Here's how the part is built. I have some questions about the finished solid (model axes, mm). Face numbers are marked on the shaded views. A direction names the side the tool comes from. Round coordinates to 2 decimals unless told otherwise and drop trailing zeros. Use a Markdown table: item, result.
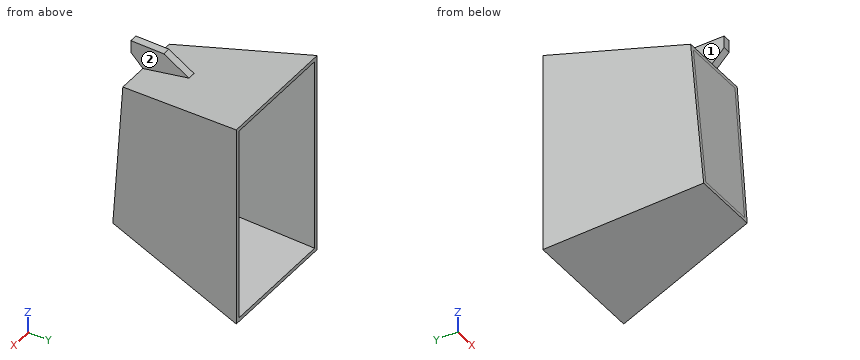
from build123d import *

# Parameters (mm, degrees)
SKETCH1_W             = 203.2
SKETCH1_H             = 336.55
BOSS_EXTRUDE4_DEPTH   = 254
BOSS_EXTRUDE4_TAPER   = 11.3
SKETCH3_W             = 190.5
SKETCH3_H             = 323.85
CUT_EXTRUDE1_DEPTH    = 247.65
CUT_EXTRUDE1_TAPER    = 11.25
CUT_EXTRUDE13_DEPTH   = 254
BOSS_EXTRUDE6_START   = 102.7176
BOSS_EXTRUDE6_DEPTH   = 12.7
BOSS_EXTRUDE7_DEPTH   = 6.35
BODY_MOVE_COPY1_ANGLE = 180
BODY_MOVE_COPY2_ANGLE = 180


with BuildPart() as part:
    # Sketch1 → Boss-Extrude4 (new body)
    with BuildSketch(Plane(origin=(0, 0, 0), x_dir=(1, 0, 0), z_dir=(0, 1, 0))):
        with Locations((-183.252356021, -34.226832461)):
            Rectangle(SKETCH1_W, SKETCH1_H)
    extrude(amount=BOSS_EXTRUDE4_DEPTH, taper=BOSS_EXTRUDE4_TAPER)

    # Sketch3 → Cut-Extrude1 (cut)
    with BuildSketch(Plane.XZ):
        with Locations((-183.252356021, 34.226832461)):
            Rectangle(SKETCH3_W, SKETCH3_H)
    extrude(amount=-CUT_EXTRUDE1_DEPTH, taper=CUT_EXTRUDE1_TAPER, mode=Mode.SUBTRACT)

    # Sketch15 → Cut-Extrude13 (cut)
    with BuildSketch(Plane(origin=(-294, 0, 0), x_dir=(0, 0, -1), z_dir=(1, 0, 0))):
        Polygon((83.293959244, 254), (-151.747624165, 254), (-159.360755409, 215.9), (87.100524866, 234.95), align=None)
    extrude(amount=CUT_EXTRUDE13_DEPTH, mode=Mode.SUBTRACT)

    # Sketch21 → Boss-Extrude6 (add)
    with BuildSketch(Plane(origin=(-294, 0, 0), x_dir=(0, 0, -1), z_dir=(1, 0, 0)).offset(BOSS_EXTRUDE6_START)):
        Polygon((-174.587017898, 139.7), (-199.360755409, 181.473734378), (-199.360755409, 235.9), (-179.360755409, 235.9), (-179.360755409, 215.9), (-159.360755409, 215.9), align=None)
        Polygon((-179.360755409, 235.9), (-179.360755409, 215.9), (-159.360755409, 215.9), align=None)
    extrude(amount=BOSS_EXTRUDE6_DEPTH)

    # Sketch22 → Boss-Extrude7 (add)
    with BuildSketch(Plane(origin=(0, 226.862283718, 17.535113426), x_dir=(1, 0, 0), z_dir=(0, 0.997026131, 0.077064226))):
        Polygon((-237.904713348, 104.947739163), (-241.71127897, -142.248670954), (-124.793433072, -142.248670954), (-128.599998694, 104.947739163), align=None)
    extrude(amount=-BOSS_EXTRUDE7_DEPTH)


with BuildPart() as part_1:
    # Body-Move/Copy1: moved
    add(part.part.rotate(Axis((0, 117.95, 34.226832461), (1, 0, 0)), BODY_MOVE_COPY1_ANGLE))


with BuildPart() as part_2:
    # Body-Move/Copy2: moved
    add(part_1.part.rotate(Axis((-183.252356021, 0, 34.226832461), (0, 1, 0)), BODY_MOVE_COPY2_ANGLE))


solid = part_2.part
1. For pin 1 Ø12 at (y, z) = (45.5, 185) entering from -X; pin 2 Ø8 at (x, y) = (-207, 113.5) entering from +Z; pin 3 Ø8 at (x, z) = (-223, 88.5) entering from +Y, each with a flat end and sliding along its axis, tell me the tip position at first contact or that it passes through.
Answer sheet:
| item | result |
|---|---|
| pin 1 | x = -187.92 |
| pin 2 | z = 178.84 |
| pin 3 | y = 21.2 |
2. I need wall thicknesses on probe 1 along Z at (x, y) = (-189.5, 78); probe 2 along X at (y, z) = (53.5, 116); probe 3 along X at (y, z) = (211.5, -18.5). Which ranges of each line are inside material? Lowest first, please. Write a range as from..to.
Answer sheet:
| item | result |
|---|---|
| probe 1 | -102.5..-96.29, 164.74..170.95 |
| probe 2 | -248.41..-242.22, -124.28..-118.1 |
| probe 3 | -279.98..-273.65, -92.86..-86.53 |
3. Which directions (+Z, -Z, +X, -X, +Y, -Y) give clear straight access to the entire face, cutting with the end or side of a thin tool? Please do the marked faces 1 and 2.
Answer sheet:
| item | result |
|---|---|
| face 1 | +Z, -X, -Y |
| face 2 | +Z, +X, -Y |
